Geometry: final body of the model. Coordinates: model frame, mm. A direction names the side the tool comes from. Coordinates: 2 decimals unless noted, no trailing zeros. Write each loop counter-clockwise with the first axis right and the second up, starting at its lowest first coordinate (ties: lowest second). Pieces come first, ordered by that corner, then holes. Notation, with made-up numbers: (-21, 77.5) -> (8, 77.5) arc R30 ccw to (8, 105.5) -> close; hole circle Ø4 at (14.5, -37.5). An arc over 180 degrees is marked (long way). Answer as a JSON object with one key per item and string values. Group by question number.
```python
from build123d import *

# Parameters (mm, degrees)
SKETCH2_W               = 129.6
SKETCH2_H               = 32
BOSS_EXTRUDE1_DEPTH     = 30
SKETCH3_W               = 2.4
SKETCH3_H               = 13.5
BOSS_EXTRUDE2_DEPTH     = 8
SKETCH4_W               = 49.5
SKETCH4_H               = 66.2
BOSS_EXTRUDE3_DEPTH     = 1.8
SKETCH5_R               = 1.75
CUT_EXTRUDE1_DEPTH      = 1.8
SKETCH6_W               = 2.35
SKETCH6_H               = 31
BOSS_EXTRUDE4_DEPTH     = 10.8
SKETCH7_W               = 17.6
SKETCH7_H               = 37.6
BOSS_EXTRUDE5_DEPTH     = 14
SKETCH8_W               = 11.5
SKETCH8_H               = 12
SKETCH8_W_2             = 12
SKETCH8_H_2             = 32.6
BOSS_EXTRUDE6_DEPTH     = 8
CUT_EXTRUDE2_DEPTH      = 8
CUT_EXTRUDE2_DEPTH_BACK = 8
SKETCH9_W               = 4.972856148
SKETCH9_H               = 7.139248924
SKETCH9_W_2             = 4.11169422
SKETCH9_H_2             = 10.539835888
SKETCH10_W              = 5.114878679
SKETCH10_H              = 27.206324026
CUT_EXTRUDE3_DEPTH      = 8
CUT_EXTRUDE4_DEPTH      = 166.599411231
CUT_EXTRUDE4_DEPTH_BACK = 129.6
SKETCH11_W              = 4
SKETCH11_H              = 32


with BuildPart() as part:
    # Sketch2 → Boss-Extrude1 (new body)
    with BuildSketch(Plane.XY):
        with Locations((64.8, 16)):
            Rectangle(SKETCH2_W, SKETCH2_H)
    extrude(amount=BOSS_EXTRUDE1_DEPTH)

    # Sketch3 → Boss-Extrude2 (add)
    with BuildSketch(Plane.ZY):
        with Locations((7.2, 16.25)):
            Rectangle(SKETCH3_W, SKETCH3_H)
        with Locations((22.8, 16.25)):
            Rectangle(SKETCH3_W, SKETCH3_H)
    extrude(amount=BOSS_EXTRUDE2_DEPTH)

    # Sketch4 → Boss-Extrude3 (add)
    with BuildSketch(Plane.ZY.offset(8)):
        with Locations((24.95, 39.1)):
            Rectangle(SKETCH4_W, SKETCH4_H)
    extrude(amount=BOSS_EXTRUDE3_DEPTH)

    # Sketch5 → Cut-Extrude1 (cut)
    with BuildSketch(Plane.ZY.offset(9.8)):
        with Locations((2.8, 69.6)):
            Circle(SKETCH5_R)
        with Locations((47.1, 69.6)):
            Circle(SKETCH5_R)
        with Locations((47.1, 8.6)):
            Circle(SKETCH5_R)
        with Locations((2.8, 8.6)):
            Circle(SKETCH5_R)
    extrude(amount=-CUT_EXTRUDE1_DEPTH, mode=Mode.SUBTRACT)

    # Sketch6 → Boss-Extrude4 (add)
    with BuildSketch(Plane(origin=(-8, 0, 0), x_dir=(0, 0, -1), z_dir=(1, 0, 0))):
        with Locations((-6.375, 49.5)):
            Rectangle(SKETCH6_W, SKETCH6_H)
        with Locations((-21.625, 49.5)):
            Rectangle(SKETCH6_W, SKETCH6_H)
    extrude(amount=BOSS_EXTRUDE4_DEPTH)

    # Sketch7 → Boss-Extrude5 (add)
    with BuildSketch(Plane(origin=(2.8, 0, 0), x_dir=(0, 0, -1), z_dir=(1, 0, 0))):
        with Locations((-14, 52.8)):
            Rectangle(SKETCH7_W, SKETCH7_H)
    extrude(amount=BOSS_EXTRUDE5_DEPTH)

    # Sketch8 → Boss-Extrude6 (add)
    with BuildSketch(Plane(origin=(-8, 0, 0), x_dir=(0, 0, -1), z_dir=(1, 0, 0))):
        with Locations((-38.75, 67.45)):
            Rectangle(SKETCH8_W, SKETCH8_H)
        with Locations((-44.95, 40.3)):
            Rectangle(SKETCH8_W_2, SKETCH8_H_2)
    extrude(amount=BOSS_EXTRUDE6_DEPTH)

    # Sketch9 → Cut-Extrude2 (cut, two sides: drawn at the far end of the back side and taken through both)
    with BuildSketch(Plane(origin=(0, 71.6, 0), x_dir=(1, 0, 0), z_dir=(0, 1, 0)).offset(-CUT_EXTRUDE2_DEPTH_BACK)):
        with Locations((-4.081901009, -38.681765119)):
            Rectangle(SKETCH9_W, SKETCH9_H)
        with BuildLine():
            Line((7.144873984, -9.259110814), (7.144873984, -17.632407274))
            ThreePointArc((7.144873984, -17.632407274), (5.446047642, -19.331233616), (3.747221299, -17.632407274))
            Line((3.747221299, -17.632407274), (3.747221299, -9.259110814))
            ThreePointArc((3.747221299, -9.259110814), (5.446047642, -7.560284471), (7.144873984, -9.259110814))
        make_face()
        with Locations((12.887635068, -13.619492602)):
            Rectangle(SKETCH9_W_2, SKETCH9_H_2)
    extrude(amount=CUT_EXTRUDE2_DEPTH + CUT_EXTRUDE2_DEPTH_BACK, mode=Mode.SUBTRACT)

    # Sketch10 → Cut-Extrude3 (cut)
    with BuildSketch(Plane.XY.offset(50.95)):
        with Locations((-4.404776722, 40.202538217)):
            Rectangle(SKETCH10_W, SKETCH10_H)
    extrude(amount=-CUT_EXTRUDE3_DEPTH, mode=Mode.SUBTRACT)

    # Sketch11 → Cut-Extrude4 (cut, two sides: drawn at the far end of the back side and taken through both)
    with BuildSketch(Plane(origin=(129.6, 0, 0), x_dir=(0, 0, -1), z_dir=(1, 0, 0)).offset(-CUT_EXTRUDE4_DEPTH_BACK)):
        with Locations((-15, 16)):
            Rectangle(SKETCH11_W, SKETCH11_H)
    extrude(amount=CUT_EXTRUDE4_DEPTH + CUT_EXTRUDE4_DEPTH_BACK, mode=Mode.SUBTRACT)


solid = part.part
```
Item 1: Mould query, pull axis Z, two halves, no side actions, for faces 1 (the flat face through (5, 63.6, 13)), 2 (the flat face through (-4, 26.599, 47)), 3 (the flat face through (-4, 16, 24)). Classes: +Z half, -Z half, draft (parallel to the pull), parting line (faces both ways), or undercut.
Item 2: Set-up query: faces 4 (the flat face through (0, 68, 39)), 5 (the flat face through (-6.962, 40, 47)), 6 (the cylindrical face through (5.48, 67.54, 19.33)). Return all of +Z, -Z, +X, -X, +Y, -Y with unobstructed straight access to the full face (end or side cutting, diameter ignored); none if empty.
Item 3: Section B-B on y = 30. Output: boundary loops of the cut face in (x, z), then the cut area to 3 significant figures.
Item 4: Section C-C on x = 69.5. Output: boundary loops of the cut face in (y, z).
Item 5: Section A-A on z = 47.1. Output: boundary loops of the cut face in (x, y), then the cut area to 3 significant figures.
Item 6: Contact query for flat-ended pins moving along their axis: pin 1 (6.5 mm diameter, centred on x = 52.5, z = 6.5, fed in from +Y); pin 2 (7.5 mm diameter, centred on x = 2.5, y = 48, fed in from -Z); pin 3 (2 mm diameter, centred on x = 48, y = 9.5, fed in from +Z); pin 4 (2 mm diameter, centred on y = 69.6, z = 47.1, fed in from +X). Output: stop coordinate, or through.
Item 7: Section D-D on z = 2.8. Output: boundary loops of the cut face in (x, y).
Item 8: Ray query, L1, parallel to Y at x = -9.35, z = 47.1; L2, parallel to Z at x = -8.5, y = 69.6; L3, parallel to Z at x = 120, y = 4.5. Return the intervals inside material, ascending. Write a range as [from, to].
Answer sheet:
{
 "1": {"face 1": "undercut", "face 2": "draft", "face 3": "+Z half"},
 "2": {"face 4": "+Z, +X, +Y, -Y", "face 5": "+Z", "face 6": "+Y"},
 "3": {"outline": "(-9.8, 0.2) -> (-8, 0.2) -> (-8, 38.95) -> (0, 38.95) -> (0, 50.95) -> (-1.85, 50.95) -> (-1.85, 42.95) -> (-6.96, 42.95) -> (-6.96, 50.95) -> (-8, 50.95) -> (-8, 49.7) -> (-9.8, 49.7) -> close; (0, 0) -> (129.6, 0) -> (129.6, 13) -> (0, 13) -> close; (0, 17) -> (129.6, 17) -> (129.6, 30) -> (0, 30) -> close", "area": "3,510 mm^2"},
 "4": {"outline": "(0, 0) -> (32, 0) -> (32, 13) -> (0, 13) -> close; (0, 17) -> (32, 17) -> (32, 30) -> (0, 30) -> close"},
 "5": {"outline": "(-9.8, 6) -> (-8, 6) -> (-8, 6.85) -> (-9.8, 6.85) -> close; (-9.8, 10.35) -> (-8, 10.35) -> (-8, 24) -> (0, 24) -> (0, 56.6) -> (-8, 56.6) -> (-8, 67.85) -> (-9.8, 67.85) -> close; (-9.8, 71.35) -> (-8, 71.35) -> (-8, 72.2) -> (-9.8, 72.2) -> close; hole (-6.96, 26.6) -> (-1.85, 26.6) -> (-1.85, 53.81) -> (-6.96, 53.81) -> close", "area": "228 mm^2"},
 "6": {"pin 1": "stops at y = 32", "pin 2": "stops at z = 5.2", "pin 3": "stops at z = 30", "pin 4": "passes through"},
 "7": {"outline": "(-9.8, 6) -> (-8, 6) -> (-8, 6.85) -> (-9.8, 6.85) -> close; (-9.8, 10.35) -> (-8, 10.35) -> (-8, 67.85) -> (-9.8, 67.85) -> close; (-9.8, 71.35) -> (-8, 71.35) -> (-8, 72.2) -> (-9.8, 72.2) -> close; (0, 0) -> (129.6, 0) -> (129.6, 32) -> (0, 32) -> close"},
 "8": {"L1": "y = [6, 6.85], [10.35, 67.85], [71.35, 72.2]", "L2": "z = [0.2, 1.05], [4.55, 45.35], [48.85, 49.7]", "L3": "z = [0, 13], [17, 30]"}
}
